Geometry check sheet. Reference: the model listing, model coordinates, mm. A direction names the side the tool comes from. Round coordinates to 2 decimals unless told otherwise and drop trailing zeros. Order: outer loops, then holes, each group sorted by start corner. A loop starts at its lowest first (then second) coordinate and runs counter-clockwise, first axis right, second up. Notation, with made-up numbers: (46.5, 11.5) -> (79.5, 11.5) arc R16 cw to (79.5, 37.5) -> close; hole circle Ø10 at (71, 16). An arc over 180 degrees is marked (long way). Use a Markdown table: item, result. Add a question column.
Item 1: Set-up check for faces 1 (the flat face through (40.697, -5.635, 3.193)), 2 (the conical face through (69.934, -17.038, 13.065)), 3 (the flat face through (0, -5, 5)): record each of +Z, -Z, +X, -X, +Y, -Y from which the full face is reachable in a straight line by a thin tool's end or side.
Item 2: Sectioned sample at A-A, the plane x = 62.5. Record the cut outline in (y, z), and give its area (3 significant figures).
Item 3: Gauge pin test, flat ends, axial feed: pin 1 Ø3.5 at (x, y) = (37, 0.5) entering from +Z; pin 2 Ø6 at (x, y) = (27.5, -11.5) entering from -Z; pin 3 Ø10 at (x, y) = (26.5, -6.5) entering from -Z. Record the tip position at first contact, or that the pin passes through.
Item 4: Material ranges on probe 1 along X at (y, z) = (-22, 5); probe 2 along Y at (x, z) = (46.5, 0); probe 3 along X at (y, z) = (17, -13), recorded low to high. Write a range as [from, to].
Item 5: Sectioned sample at C-C, the plane x = 43. Record the cut outline in (y, z), and give its area (3 significant figures).
Item 6: Mould release check, pull along Y, two halves, no side actions. Record for faces 4 (the flat face through (40.697, 5.635, -3.193)), 5 (the flat face through (41, 0, -6.477)), 6 (the conical face through (44.385, -4.667, 21.017)), 7 (the flat face through (82.55, -5, 5)): pulls with the +Y half, pulls with the -Y half, needs draft (parallel to the pull), parting line crosses it, or undercut.
from build123d import *

# Parameters (mm, degrees)
SKETCH1_W          = 82.55
SKETCH1_H          = 25.4
CUT_EXTRUDE1_DEPTH = 83.55


with BuildPart() as part:
    # Sketch1 → Revolve1 (revolve)
    with BuildSketch(Plane.XY):
        with Locations((41.275, 12.7)):
            Rectangle(SKETCH1_W, SKETCH1_H)
    revolve(axis=Axis((0, 0, 0), (-1, 0, 0)))

    # Sketch2 → Cut-Revolve1 (revolve, cut)
    with BuildSketch(Plane.XY):
        with BuildLine():
            Line((5.194846373, 25.4), (6.496948681, 21.270259087))
            ThreePointArc((6.496948681, 21.270259087), (9.525, 19.05), (12.553051319, 21.270259087))
            Line((12.553051319, 21.270259087), (13.855153627, 25.4))
            Line((13.855153627, 25.4), (5.194846373, 25.4))
        make_face()
        with BuildLine():
            Line((36.944846373, 25.4), (38.246948681, 21.270259087))
            ThreePointArc((38.246948681, 21.270259087), (41.275, 19.05), (44.303051319, 21.270259087))
            Line((44.303051319, 21.270259087), (45.605153627, 25.4))
            Line((45.605153627, 25.4), (36.944846373, 25.4))
        make_face()
        with BuildLine():
            Line((68.694846373, 25.4), (69.996948681, 21.270259087))
            ThreePointArc((69.996948681, 21.270259087), (73.025, 19.05), (76.053051319, 21.270259087))
            Line((76.053051319, 21.270259087), (77.355153627, 25.4))
            Line((77.355153627, 25.4), (68.694846373, 25.4))
        make_face()
    revolve(axis=Axis((0, 0, 0), (-1, 0, 0)), mode=Mode.SUBTRACT)

    # Sketch3 → Cut-Extrude1 (cut, through all)
    with BuildSketch(Plane.ZY):
        Polygon((0, 7.478995387), (-6.477, 3.739497694), (-6.477, -3.739497694), (0, -7.478995387), (6.477, -3.739497694), (6.477, 3.739497694), align=None)
    extrude(amount=-CUT_EXTRUDE1_DEPTH, mode=Mode.SUBTRACT)


solid = part.part
Found:
| question | item | result |
|---|---|---|
| 1 | face 1 | +X, -X |
| 1 | face 2 | none |
| 1 | face 3 | +Z, -Z, -X, +Y, -Y |
| 2 | outline | circle Ø50.8 at (0, 0); hole (-7.48, 0) -> (-3.74, -6.48) -> (3.74, -6.48) -> (7.48, 0) -> (3.74, 6.48) -> (-3.74, 6.48) -> close |
| 2 | area | 1,880 mm2 |
| 3 | pin 1 | stops at z = 25.4 |
| 3 | pin 2 | stops at z = -23.94 |
| 3 | pin 3 | stops at z = -25.36 |
| 4 | probe 1 | x = [0, 6.09], [12.96, 37.84], [44.71, 69.59], [76.46, 82.55] |
| 4 | probe 2 | y = [-25.4, -7.48], [7.48, 25.4] |
| 4 | probe 3 | x = [0, 6.46], [12.59, 38.21], [44.34, 69.96], [76.09, 82.55] |
| 5 | outline | circle Ø39.12 at (0, 0); hole (-7.48, 0) -> (-3.74, -6.48) -> (3.74, -6.48) -> (7.48, 0) -> (3.74, 6.48) -> (-3.74, 6.48) -> close |
| 5 | area | 1,060 mm2 |
| 6 | face 4 | undercut |
| 6 | face 5 | undercut |
| 6 | face 6 | parting line crosses it |
| 6 | face 7 | needs draft |
